Check sheet for the modelled part. Datum: model origin and axes. Units: mm. Face numbers are marked on the shaded views. A direction names the side the tool comes from. Coordinates: 2 decimals unless noted, no trailing zeros. Write each loop counter-clockwise with the first axis right and the second up, starting at its lowest first coordinate (ties: lowest second). Pieces come first, ordered by that corner, then holes. Notation, with made-up numbers: (41, 63.25) -> (57, 63.25) arc R31 ccw to (57, 96.25) -> close; hole circle Ø2 at (41.5, 19.25). An arc over 180 degrees is marked (long way). Put each result on its own line as item: value.
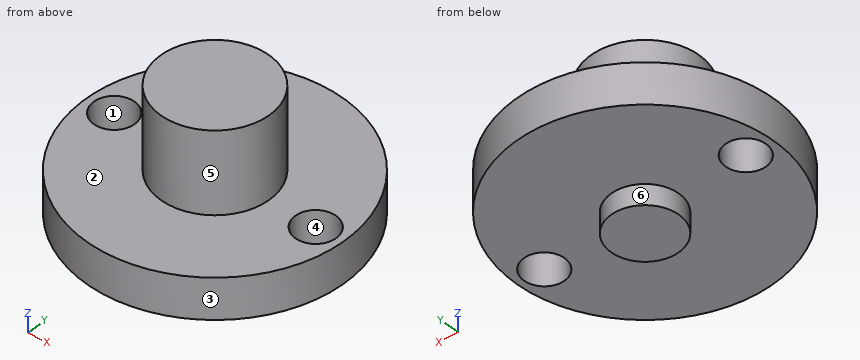
```python
from build123d import *

# Parameters (mm, degrees)
CROQUIS1_R              = 9.5
SALIENTE_EXTRUIR1_DEPTH = 3
CROQUIS2_R              = 4
SALIENTE_EXTRUIR2_DEPTH = 6
CROQUIS3_R              = 2.5
SALIENTE_EXTRUIR3_DEPTH = 1.5
CROQUIS4_R              = 1.5
CORTAR_EXTRUIR1_DEPTH   = 15.71393897


with BuildPart() as part:
    # Croquis1 → Saliente-Extruir1 (new body)
    with BuildSketch(Plane.XY):
        Circle(CROQUIS1_R)
    extrude(amount=SALIENTE_EXTRUIR1_DEPTH)

    # Croquis2 → Saliente-Extruir2 (add)
    with BuildSketch(Plane.XY.offset(3)):
        Circle(CROQUIS2_R)
    extrude(amount=SALIENTE_EXTRUIR2_DEPTH)

    # Croquis3 → Saliente-Extruir3 (add)
    with BuildSketch(Plane(origin=(0, 0, 0), x_dir=(-1, 0, 0), z_dir=(0, 0, -1))):
        Circle(CROQUIS3_R)
    extrude(amount=SALIENTE_EXTRUIR3_DEPTH)

    # Croquis4 → Cortar-Extruir1 (cut, through all)
    with BuildSketch(Plane.XY.offset(3)):
        with Locations((-7.5, 0)):
            Circle(CROQUIS4_R)
        with Locations((7.5, 0)):
            Circle(CROQUIS4_R)
    extrude(amount=-CORTAR_EXTRUIR1_DEPTH, mode=Mode.SUBTRACT)


solid = part.part
```
Q1. Cross-section at D-D (y = -3.25). Record the cut outline in (x, z), plus the area to 3 significant figures.
Recorded:
outline: (-8.93, 0) -> (8.93, 0) -> (8.93, 3) -> (2.33, 3) -> (2.33, 9) -> (-2.33, 9) -> (-2.33, 3) -> (-8.93, 3) -> close
area: 81.5 mm2
Q2. Tool access check on the marked faces 4, 5 and 6. Record the directions out of +Z, -Z, +X, -X, +Y, -Y that give a thin tool (end or side, any length) a straight path to the whole face; none if there is none.
Recorded:
face 4: +Z, -Z
face 5: +Z
face 6: -Z
Q3. Cross-section at C-C (x = -7.5). Record the cut outline in (y, z), plus the area to 3 significant figures.
Recorded:
outline: (-5.83, 0) -> (-1.5, 0) -> (-1.5, 3) -> (-5.83, 3) -> close; (1.5, 0) -> (5.83, 0) -> (5.83, 3) -> (1.5, 3) -> close
area: 26.0 mm2
Q4. Cross-section at A-A (y = 0). Record the cut outline in (x, z).
Recorded:
outline: (-9.5, 0) -> (-9, 0) -> (-9, 3) -> (-9.5, 3) -> close; (-6, 0) -> (-2.5, 0) -> (-2.5, -1.5) -> (2.5, -1.5) -> (2.5, 0) -> (6, 0) -> (6, 3) -> (4, 3) -> (4, 9) -> (-4, 9) -> (-4, 3) -> (-6, 3) -> close; (9, 0) -> (9.5, 0) -> (9.5, 3) -> (9, 3) -> close
Q5. Cross-section at B-B (x = 0). Record the cut outline in (y, z).
Recorded:
outline: (-9.5, 0) -> (-2.5, 0) -> (-2.5, -1.5) -> (2.5, -1.5) -> (2.5, 0) -> (9.5, 0) -> (9.5, 3) -> (4, 3) -> (4, 9) -> (-4, 9) -> (-4, 3) -> (-9.5, 3) -> close
Q6. Mould release check, pull along Y, two halves, no side actions. Record for the marked faces 1, 2 and 3: released by +Y, released by -Y, zero draft, split by the parting line, or undercut.
Recorded:
face 1: undercut
face 2: zero draft
face 3: split by the parting line
Q7. Material ranges on line 1 along Y through (x, z) = (7.5, 1.4); line 2 along Z through (x, y) = (-8, -4.75); line 3 along X through (y, z) = (-1, 6.5), recorded low to high.
Recorded:
line 1: y = -5.83 to -1.5, 1.5 to 5.83
line 2: z = 0 to 3
line 3: x = -3.87 to 3.87
Q8. Depth check by flat-ended pin: P1, Ø3.5, axis at x = -7.5, y = 0, coming from the -Z side; P2, Ø1, axis at x = -3, z = 2.5, coming from the -Y side; P3, Ø5, axis at x = -3.5, z = 7.5, coming from the +Y side. Enter the tip coordinate at first touch or a pass-through.
Recorded:
P1: stops at z = 0
P2: stops at y = -9.17
P3: stops at y = 3.87
